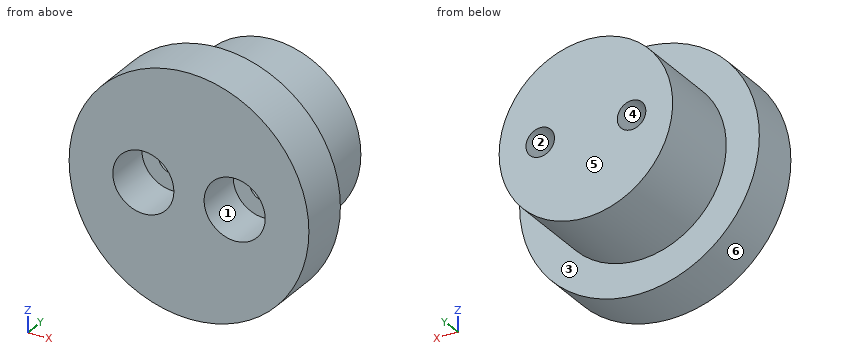
from build123d import *

# Parameters (mm, degrees)
SKETCH2_R           = 7.6
SKETCH2_R_2         = 1.25
BOSS_EXTRUDE2_DEPTH = 10.15
SKETCH3_R           = 10.5
SKETCH3_R_2         = 1.25
BOSS_EXTRUDE3_DEPTH = 2.5
SKETCH4_R           = 2.675
CUT_EXTRUDE1_DEPTH  = 2.15
SKETCH5_R           = 10.5
SKETCH5_R_2         = 2.675
BOSS_EXTRUDE4_DEPTH = 2


with BuildPart() as part:
    # Sketch2 → Boss-Extrude2 (new body)
    with BuildSketch(Plane(origin=(0, 0, 0), x_dir=(1, 0, 0), z_dir=(0, 1, 0))):
        Circle(SKETCH2_R)
        with Locations((4, 0)):
            Circle(SKETCH2_R_2, mode=Mode.SUBTRACT)
        with Locations((-4, 0)):
            Circle(SKETCH2_R_2, mode=Mode.SUBTRACT)
    extrude(amount=BOSS_EXTRUDE2_DEPTH)

    # Sketch3 → Boss-Extrude3 (add)
    with BuildSketch(Plane(origin=(0, 0, 0), x_dir=(1, 0, 0), z_dir=(0, 1, 0))):
        Circle(SKETCH3_R)
        with Locations((-4, 0)):
            Circle(SKETCH3_R_2, mode=Mode.SUBTRACT)
        with Locations((4, 0)):
            Circle(SKETCH3_R_2, mode=Mode.SUBTRACT)
    extrude(amount=BOSS_EXTRUDE3_DEPTH)

    # Sketch4 → Cut-Extrude1 (cut)
    with BuildSketch(Plane.XZ):
        with Locations((4, 0)):
            Circle(SKETCH4_R)
        with Locations((-4, 0)):
            Circle(SKETCH4_R)
    extrude(amount=-CUT_EXTRUDE1_DEPTH, mode=Mode.SUBTRACT)

    # Sketch5 → Boss-Extrude4 (add)
    with BuildSketch(Plane.XZ):
        Circle(SKETCH5_R)
        with Locations((-4, 0)):
            Circle(SKETCH5_R_2, mode=Mode.SUBTRACT)
        with Locations((4, 0)):
            Circle(SKETCH5_R_2, mode=Mode.SUBTRACT)
    extrude(amount=BOSS_EXTRUDE4_DEPTH)


solid = part.part
Verification items for the finished model (mm, model axes). Face numbers are marked on the shaded views. A direction names the side the tool comes from. Coordinates: 2 decimals unless noted, no trailing zeros. Order: outer loops, then holes, each group sorted by start corner. A loop starts at its lowest first (then second) coordinate and runs counter-clockwise, first axis right, second up.
Item 1: Depth check by flat-ended pin: pin 1 (6 mm diameter, centred on y = 8.5, z = -6.5, fed in from +X); pin 2 (3 mm diameter, centred on x = 4, z = 0, fed in from -Y); pin 3 (5 mm diameter, centred on y = 7.5, z = -5.5, fed in from +X); pin 4 (2 mm diameter, centred on x = -4, z = 0, fed in from -Y). Enter the tip coordinate at first touch or a pass-through.
Filled in:
pin 1: stops at x = 6.75
pin 2: stops at y = 2.15
pin 3: stops at x = 6.98
pin 4: passes through
Item 2: Access from +Z, -Z, +X, -X, +Y, -Y to the whole of each face (thin tool, end or side, straight path). Record for the marked faces 1, 2 and 3.
Filled in:
face 1: -Y
face 2: +Y, -Y
face 3: +Y
Item 3: Release check for a two-part mould opening along Z. For the marked faces 4, 5 and 6 record: +Z half, -Z half, draft (parallel to the pull), parting line (faces both ways), or undercut.
Filled in:
face 4: undercut
face 5: draft
face 6: parting line
Item 4: Section check A-A, the plane z = 0. Enter the section's corners in (x, y) (3 decimals), then the cut area to 3 significant figures.
Filled in:
outline: (-10.5, -2) - (-6.675, -2) - (-6.675, 2.15) - (-5.25, 2.15) - (-5.25, 10.15) - (-7.6, 10.15) - (-7.6, 2.5) - (-10.5, 2.5) - close; (-2.75, 2.15) - (-1.325, 2.15) - (-1.325, -2) - (1.325, -2) - (1.325, 2.15) - (2.75, 2.15) - (2.75, 10.15) - (-2.75, 10.15) - close; (5.25, 2.15) - (6.675, 2.15) - (6.675, -2) - (10.5, -2) - (10.5, 2.5) - (7.6, 2.5) - (7.6, 10.15) - (5.25, 10.15) - close
area: 126 mm2
Item 5: Section check D-D, the plane y = 0. Enter the section's corners in (x, z) (3 decimals), then the cut area to 3 significant figures.
Filled in:
outline: circle Ø21 at (0, 0); hole circle Ø5.35 at (-4, 0); hole circle Ø5.35 at (4, 0)
area: 301 mm2
Item 6: Material ranges on L1, parallel to X at y = 4.5, z = 0; L2, parallel to X at y = -0.5, z = -0.5; L3, parallel to Y at x = -7.25, z = 3.5, recorded low to high.
Filled in:
L1: x = -7.6 to -5.25, -2.75 to 2.75, 5.25 to 7.6
L2: x = -10.49 to -6.63, -1.37 to 1.37, 6.63 to 10.49
L3: y = -2 to 2.5
Item 7: Section check C-C, the plane x = 0. Enter the section's corners in (y, z).
Filled in:
outline: (-2, -10.5) - (2.5, -10.5) - (2.5, -7.6) - (10.15, -7.6) - (10.15, 7.6) - (2.5, 7.6) - (2.5, 10.5) - (-2, 10.5) - close
Item 8: Section check B-B, the plane x = 4. Enter the section's corners in (y, z) (3 decimals), then the cut area to 3 significant figures.
Filled in:
outline: (-2, -9.708) - (2.5, -9.708) - (2.5, -6.462) - (10.15, -6.462) - (10.15, -1.25) - (2.15, -1.25) - (2.15, -2.675) - (-2, -2.675) - close; (-2, 2.675) - (2.15, 2.675) - (2.15, 1.25) - (10.15, 1.25) - (10.15, 6.462) - (2.5, 6.462) - (2.5, 9.708) - (-2, 9.708) - close
area: 144 mm2
